Could you check a few things on this model? Use its own coordinates, in mm. A direction names the side the tool comes from. Coordinates: 2 decimals unless noted, no trailing zeros. Loops run counter-clockwise (first coordinate to the right, second up) from the corner with the lowest first, then second, coordinate; pieces in that order, holes last.
Autodesk Inventor part; units mm, degrees
ref_plane "bolt_XY" through (0, 0, 0) normal (1, 0, 0) x (0, 0, -1)
ref_plane "bolt_YZ" through (0, 0, 0) normal (0, 0, -1) x (0, 1, 0)
ref_plane "bolt_ZX" through (0, 0, 0) normal (0, 1, 0) x (1, 0, 0)
sketch "Sketch_8" plane through (0, 0, 0) normal (0, 0, 1) x (1, 0, 0)
  line L0 (10, 0) -> (-5, 0)
  line L1 (-5, 0) -> (-5, 3.9613)
  line L2 (-5, 3.9613) -> (-4.5, 4.25)
  line L3 (-4.5, 4.25) -> (0, 4.25)
  line L4 (0, 4.25) -> (0, 2.7)
  arc A0 (0, 2.7) -> (0.2, 2.5) centre (0.2, 2.7) ccw
  line L5 (0.2, 2.5) -> (9.5095, 2.5)
  line L6 (9.5095, 2.5) -> (10, 2.0095)
  line L7 (10, 2.0095) -> (10, 0)
  line L8 (10, 0) -> (-5, 0)
revolve "Revolution1" add sketch "Sketch_8" angle 360 about axis through (10, 0, 0) along (1, 0, 0)
thread "Thread1"
sketch "Sketch2" plane through (-5, 0, 0) normal (-1, 0, 0) x (0, 0, 1)
  point P0 (0, 0)
hole "Hole1" at (-5, 0, 0) direction (1, 0, 0) diameter 4 depth 2.5 tip angle 120
sketch "Sketch_3" plane through (-5, 0, 0) normal (1, 0, 0) x (0, 0, -1)
  line L0 (-2, -1.1547) -> (0, -2.3094)
  line L1 (0, -2.3094) -> (2, -1.1547)
  line L2 (2, -1.1547) -> (2, 1.1547)
  line L3 (2, 1.1547) -> (0, 2.3094)
  line L4 (0, 2.3094) -> (-2, 1.1547)
  line L5 (-2, 1.1547) -> (-2, -1.1547)
extrude "Extrusion1" cut sketch "Sketch_3" along normal blind 2.5
ref_plane "bolt_XY" through (0, 0, 0) normal (1, 0, 0) x (0, 0, -1)
ref_plane "bolt_YZ" through (0, 0, 0) normal (0, 0, -1) x (0, 1, 0)
ref_plane "bolt_ZX" through (0, 0, 0) normal (0, 1, 0) x (1, 0, 0)
ref_plane "nut_XY" through (10, 0, 0) normal (1, 0, 0) x (0, 0, -1)
ref_plane "nut_YZ" through (10, 0, 0) normal (0, 0, -1) x (0, 1, 0)
ref_plane "nut_ZX" through (10, 0, 0) normal (0, 1, 0) x (1, 0, 0)
properties part number "CBM5-10"
1) We'd pull the mould along Z, two halves only. Please class faces 1 (the flat face through (-3.77, 1.74, 0.99)), 2 (the flat face through (10, 0, 0)), 3 (the cylindrical face through (4.92, -0.54, -2.44)): released by +Z, released by -Z, zero draft, split by the parting line, or undercut.
2) Imagine slicing it at B-B on x = 2.5. List the corners of the cut face in (y, z) for me.
3) Will these pins go through, and if not, where does the flat tip stop? pin 1 (3 mm diameter, centred on x = -1.5, y = 2.5, fed in from +Z); pin 2 (1.5 mm diameter, centred on y = -2.5, z = 2.5, fed in from +X); pin 3 (0.5 mm diameter, centred on y = 1, z = -1.5, fed in from -X).
4) For faces 4 (the flat face through (0, 0, -3)), 5 (the flat face through (-4, 0, -2)), 6 (the flat face through (-5, -2, 1)), which set-ups out of +Z, -Z, +X, -X, +Y, -Y let a thin tool reach every point of the face, with its end or its side?
5) Imagine slicing it at A-A on x = -3.25. List the corners of the cut face in (y, z) for me, plus the area to 3 significant figures.
6) If I drill on L1, parallel to X at y = -3, z = 1.5; L2, parallel to Z at x = -3.25, y = -1; L3, parallel to Z at x = 7, y = -1.5, over which ranges is the centre line in solid material (lowest first)?
Solved:
1. face 1: undercut
1. face 2: zero draft
1. face 3: split by the parting line
2. outline: circle Ø5 at (0, 0)
3. pin 1: stops at z = 4.13
3. pin 2: stops at x = 0
3. pin 3: stops at x = -2.5
4. face 4: +X
4. face 5: -X
4. face 6: +Z, -Z, -X, +Y, -Y
5. outline: circle Ø8.5 at (0, 0); hole (-2.31, 0) - (-1.15, -2) - (1.15, -2) - (2.31, 0) - (1.15, 2) - (-1.15, 2) - close
5. area: 42.9 mm2
6. L1: x = -5 to 0
6. L2: z = -4.13 to -2, 2 to 4.13
6. L3: z = -2 to 2
